from build123d import *

# Parameters (mm, degrees)
F0_W     = 15
F0_H     = 20
F1_DEPTH = 15
F2_F1_R  = 5
F2_F2_R  = 5
F2_F3_R  = 5
F2_F4_R  = 5
F2_F5_R  = 5


# Not quite as in the source:
# - a feature of the source that left no trace in its solid (it failed there, or was rolled back) is left out
# - a feature names something its author has since deleted; it is built from what else it names


with BuildPart() as f1:
    # F0 (on Front) → F1 (new body)
    with BuildSketch(Plane.XZ):
        with BuildLine():
            add(Edge.make_bspline(
                [(80, 15), (90.0562568152, 15), (96.9973913685, 23.3758884073), (96.9973913685, 31.4775960116)],
                knots=[0, 0, 0, 0, 23.6732440459, 23.6732440459, 23.6732440459, 23.6732440459], degree=3))
            Line((80, 15), (79.8229584098, 0))
            add(Edge.make_bspline(
                [(111.9973913685, 31.4775960116), (111.9973913685, 15), (96.9973913685, 0), (79.8229584098, 0)],
                knots=[0, 0, 0, 0, 45.0114783904, 45.0114783904, 45.0114783904, 45.0114783904], degree=3))
            Line((111.9973913685, 31.4775960116), (96.9973913685, 31.4775960116))
        make_face()
        with Locations((104.4973913685, 41.4775960116)):
            Rectangle(F0_W, F0_H)
        Polygon((80, 15), (0, 15), (0, 0), (79.8229584098, 0), align=None)
    extrude(amount=F1_DEPTH)

    # F2: fillet of radius 5 on 20 edges, made by hand

    # F2_f1
    f2_f1_edges = [f1.edges().sort_by_distance(p)[0] for p in [
        (92.2697919899, 0, 20.2006576542),
        (96.9973913685, 0, 41.4775960116),
        (40, 0, 15),
    ]]
    fillet(f2_f1_edges, radius=F2_F1_R)

    # F2_f2
    f2_f2_edges = [f1.edges().sort_by_distance(p)[0] for p in [
        (92.2697919899, -15, 20.2006576542),
        (96.9973913685, -15, 41.4775960116),
        (40, -15, 15),
    ]]
    fillet(f2_f2_edges, radius=F2_F2_R)

    # F2_f3
    f2_f3_edges = [f1.edges().sort_by_distance(p)[0] for p in [
        (96.9973913685, -7.5, 51.4775960116),
    ]]
    fillet(f2_f3_edges, radius=F2_F3_R)

    # F2_f4
    f2_f4_edges = [f1.edges().sort_by_distance(p)[0] for p in [
        (111.9973913685, -7.5, 51.4775960116),
    ]]
    fillet(f2_f4_edges, radius=F2_F4_R)

    # F2_f5
    f2_f5_edges = [f1.edges().sort_by_distance(p)[0] for p in [
        (0, -7.5, 0),
    ]]
    fillet(f2_f5_edges, radius=F2_F5_R)


solid = f1.part
Could you check a few things on this model? Use its own coordinates, in mm. A direction names the side the tool comes from. Give positions to 0.01 mm unless a question says otherwise; leave off trailing zeros. Order: outer loops, then holes, each group sorted by start corner. A loop starts at its lowest first (then second) coordinate and runs counter-clockwise, first axis right, second up.
1. Suppose I cut it at B-B (z = 38.5). Write out the boundary of the cut face in (x, y), plus the area to 3 significant figures.
Answers below:
outline: (97, -10) arc R5 ccw to (102, -15) - (107, -15) arc R5 ccw to (112, -10) - (112, -5) arc R5 ccw to (107, 0) - (102, 0) arc R5 ccw to (97, -5) - close
area: 204 mm2
2. I need wall thicknesses on L1, parallel to Z at x = 32.5, y = -6.25; L2, parallel to Z at x = 36.5, y = -0.75; L3, parallel to X at y = -2, z = 10.5. Which ranges of each line are inside material? Lowest first, please.
Answers below:
L1: z = 0 to 15
L2: z = 2.37 to 12.63
L3: x = 1.03 to 101.88
3. Suppose I cut it at A-A (x = 35). Write out the boundary of the cut face in (y, z).
Answers below:
outline: (-15, 5) arc R5 ccw to (-10, 0) - (-5, 0) arc R5 ccw to (0, 5) - (0, 10) arc R5 ccw to (-5, 15) - (-10, 15) arc R5 ccw to (-15, 10) - close
4. Which directions (+Z, -Z, +X, -X, +Y, -Y) give clear straight access to the entire face, cutting with the end or side of a thin tool? Please do faces 1 (the flat face through (96.997, -7, 39)), 2 (the cylindrical face through (98.423, -13.496, 39.083)), 3 (the flat face through (111.997, -7, 39)).
Answers below:
face 1: +Z, -X, +Y, -Y
face 2: +Z, -X, -Y
face 3: +Z, -Z, +X, +Y, -Y
5. For pin 1 (1.5 mm diameter, centred on x = 53.5, y = -6.5, fed in from +Z); pin 2 (2 mm diameter, centred on x = 74.5, z = 13, fed in from +Y); pin 3 (4 mm diameter, centred on y = -8, z = 36.5, fed in from -X), each with a flat end and sliding along its axis, tell me the tip position at first contact or that it passes through.
Answers below:
pin 1: stops at z = 15
pin 2: stops at y = -0.42
pin 3: stops at x = 97
